Read the model definition and answer for the solid it produces. Units are mm, in the model's axes. A direction names the side the tool comes from. Coordinates: 2 decimals unless noted, no trailing zeros. Order: outer loops, then holes, each group sorted by start corner. A loop starts at its lowest first (then second) coordinate and runs counter-clockwise, first axis right, second up. Notation, with made-up numbers: M -24.75,-38 L 29.25,-38 A19 ccw 29.25,-1 Z; hole C -4,19.25 d5. An arc over 180 degrees is marked long. Put each result on its own line as item: value.
from build123d import *

# Parameters (mm, degrees)
F0_R     = 3.175
F1_DEPTH = 59.69
F2_R     = 5.08
F3_R     = 2.5527
F4_DEPTH = 18.4414
F5_R     = 5.08


with BuildPart() as f1:
    # F0 (on Front) → F1 (new body)
    with BuildSketch(Plane.XZ):
        with BuildLine():
            Line((0, 14.925174), (0, 0))
            Line((0, 0), (18.4404, 0))
            Line((18.4404, 0), (18.4404, 91.44))
            Line((18.4404, 91.44), (0, 91.44))
            Line((0, 91.44), (0, 76.514826))
            ThreePointArc((0, 76.514826), (13.7922, 45.72), (0, 14.925174))
        make_face()
        with Locations((5.08, 7.62)):
            Circle(F0_R, mode=Mode.SUBTRACT)
        with Locations((5.08, 83.82)):
            Circle(F0_R, mode=Mode.SUBTRACT)
    extrude(amount=F1_DEPTH)

    # F2
    f2_edges = [f1.edges().sort_by_distance(p)[0] for p in [
        (0, -29.845, 91.44),
        (0, -29.845, 0),
    ]]
    fillet(f2_edges, radius=F2_R)

    # F3 (on face) → F4 (cut, through all)
    with BuildSketch(Plane.YZ.offset(18.4404)):
        with Locations((-47.625, 59.944)):
            Circle(F3_R)
        with Locations((-12.065, 59.944)):
            Circle(F3_R)
        with Locations((-29.845, 31.496)):
            Circle(F3_R)
        with BuildLine():
            Line((-12.065, 91.44), (-47.625, 91.44))
            Line((-47.625, 91.44), (-47.625, 76.454))
            ThreePointArc((-47.625, 76.454), (-45.765128, 71.963872), (-41.275, 70.104))
            Line((-41.275, 70.104), (-18.415, 70.104))
            ThreePointArc((-18.415, 70.104), (-13.924872, 71.963872), (-12.065, 76.454))
            Line((-12.065, 76.454), (-12.065, 91.44))
        make_face()
        with BuildLine():
            Line((-47.625, 14.986), (-47.625, 0))
            Line((-47.625, 0), (-12.065, 0))
            Line((-12.065, 0), (-12.065, 14.986))
            ThreePointArc((-12.065, 14.986), (-13.924872, 19.476128), (-18.415, 21.336))
            Line((-18.415, 21.336), (-41.275, 21.336))
            ThreePointArc((-41.275, 21.336), (-45.765128, 19.476128), (-47.625, 14.986))
        make_face()
        with BuildLine():
            Line((-10.178521, 41.924013), (-27.958521, 61.644822))
            ThreePointArc((-27.958521, 61.644822), (-29.845, 62.484), (-31.731479, 61.644822))
            Line((-31.731479, 61.644822), (-49.511479, 41.924013))
            ThreePointArc((-49.511479, 41.924013), (-49.891828, 39.07729), (-47.373991, 37.695624))
            Line((-47.373991, 37.695624), (-12.316009, 37.695624))
            Line((-12.316009, 37.695624), (-11.813991, 37.695624))
            ThreePointArc((-11.813991, 37.695624), (-9.696027, 39.306912), (-10.178521, 41.924013))
        make_face()
        with BuildLine():
            ThreePointArc((-12.316009, 37.695624), (-12.065, 37.683191), (-11.813991, 37.695624))
            Line((-11.813991, 37.695624), (-12.316009, 37.695624))
        make_face()
    extrude(amount=-F4_DEPTH, mode=Mode.SUBTRACT)

    # F5
    f5_edges = [f1.edges().sort_by_distance(p)[0] for p in [
        (18.4404, -53.6575, 91.44),
        (18.4404, -6.0325, 91.44),
        (18.4404, -53.6575, 0),
        (18.4404, -6.0325, 0),
    ]]
    fillet(f5_edges, radius=F5_R)


solid = f1.part
Q1. A tool of negligible diameter and unlimited length cuts with its end or side. For faces 5 (the face through (16.992, -53.742, 1.528)), 6 (the face through (11.424, -13.975, 71.915)), 7 (the face through (15.445, -38.521, 54.114)), 8 (the face through (9, -6, 0)), 9 (the face through (9, -12.065, 7)), from which of +Z, -Z, +X, -X, +Y, -Y can it reach the whole face along a straight path? Write none if from no direction.
Answers below:
face 5: -Z, +X, +Y, -Y
face 6: +Z, +X, -X
face 7: +X, -X
face 8: -Z, +X, -X, +Y, -Y
face 9: -Z, +X, -X
Q2. For a pull along X with two mould halves and no side action, classify faces 1 (the face through (11.42, -13.88, 19.43)), 2 (the face through (4.39, -5.95, 80.72)), 3 (the face through (4.39, -5.95, 4.52)), 4 (the face through (18.44, -29, 36)) as +X half, -X half, draft (parallel to the pull), parting line (faces both ways), or undercut.
Answers below:
face 1: draft
face 2: undercut
face 3: undercut
face 4: +X half
Q3. Find section D-D on y = -54.5. Write down the section's boundary in (x, z) (3 decimals), plus the area to 3 significant figures.
Answers below:
outline: M 0,5.08 A5.08 ccw 5.08,0 L 13.36,0 A5.08 ccw 18.44,5.08 L 18.44,86.36 A5.08 ccw 13.36,91.44 L 5.08,91.44 A5.08 ccw 0,86.36 L 0,76.515 A41.275 cw 0,14.925 Z; hole C 5.08,7.62 d6.35; hole C 5.08,83.82 d6.35
area: 1,010 mm^2
Q4. Find section B-B on y = -13.5. Write down the section's boundary in (x, z) (3 decimals).
Answers below:
outline: M 3.982,19.007 L 18.44,19.007 L 18.44,37.696 L 13.005,37.696 A41.275 cw Z; M 3.982,72.433 A41.275 cw 10.422,62.055 L 18.44,62.055 L 18.44,72.433 Z; M 11.975,57.833 A41.275 cw 13.792,45.608 L 18.44,45.608 L 18.44,57.833 Z
Q5. Find section A-A on z = 83.82. Write down the section's boundary in (x, y) (3 decimals), plus the area to 3 significant figures.
Answers below:
outline: M 0,-59.69 L 1.905,-59.69 L 1.905,-47.625 L 0,-47.625 Z; M 0,-12.065 L 1.905,-12.065 L 1.905,0 L 0,0 Z; M 8.255,-59.69 L 18.44,-59.69 L 18.44,-47.625 L 8.255,-47.625 Z; M 8.255,-12.065 L 18.44,-12.065 L 18.44,0 L 8.255,0 Z
area: 292 mm^2
Q6. Consider line 1 along Y through (x, z) = (9.75, 86.5) (3 decimals); line 2 along Z through (x, y) = (7.75, -51); line 3 along Z through (x, y) = (5.08, -3.5) (3 decimals). Determine where each line is inside the solid, lowest interval first.
Answers below:
line 1: y = -59.69 to -47.625, -12.065 to 0
line 2: z = 0 to 5.9, 9.34 to 24.22, 67.22 to 82.1, 85.54 to 91.44
line 3: z = 0 to 4.445, 10.795 to 20.357, 71.083 to 80.645, 86.995 to 91.44
Q7. Find section C-C on x = 16.5. Write down the section's boundary in (y, z) (3 decimals).
Answers below:
outline: M -59.69,1.086 L -47.625,1.086 L -47.625,14.986 A6.35 cw -41.275,21.336 L -18.415,21.336 A6.35 cw -12.065,14.986 L -12.065,1.086 L 0,1.086 L 0,90.354 L -12.065,90.354 L -12.065,76.454 A6.35 cw -18.415,70.104 L -41.275,70.104 A6.35 cw -47.625,76.454 L -47.625,90.354 L -59.69,90.354 Z; hole C -47.625,59.944 d5.105; hole M -49.511,41.924 A2.54 ccw -47.374,37.696 L -12.316,37.696 A2.54 ccw -11.814,37.696 A2.54 ccw -10.179,41.924 L -27.959,61.645 A2.54 ccw -31.731,61.645 Z; hole C -29.845,31.496 d5.105; hole C -12.065,59.944 d5.105
Q8. Given pin 1 (4 mm diameter, centred on x = 9, y = -32, fed in from -Z); pin 2 (5 mm diameter, centred on x = 5.08, z = 83.82, fed in from -Y); pin 3 (1 mm diameter, centred on y = -25.5, z = 70.5, fed in from -X); pin 4 (4 mm diameter, centred on y = -39, z = 66, fed in from -X), each flat-ended and moving along its own axis, determine where each tip first touches the part or whether it passes through.
Answers below:
pin 1: stops at z = 21.34
pin 2: passes through
pin 3: stops at x = 5.82
pin 4: stops at x = 7.26
